Autodesk Inventor part; units mm, degrees
ref_plane "Work Plane1" through (94.25, -2.5, 0) normal (1, 0, 0) x (0, 0, -1)
ref_plane "YZ Plane" through (0, 0, 0) normal (1, 0, 0) x (0, 1, 0)
ref_plane "XZ Plane" through (0, 0, 0) normal (0, 1, 0) x (-1, 0, 0)
sketch "Sketch2" plane through (0, 0, 0) normal (0, 0, 1) x (1, 0, 0)
  line L0 (-99.5, 2.5) -> (99.5, 2.5)
  line L1 (99.5, 2.5) -> (99.5, -2.5)
  line L2 (99.5, -2.5) -> (-99.5, -2.5)
  line L3 (-99.5, -2.5) -> (-99.5, 2.5)
  point P0 (0, 0)
  dimension "d1" = 199
  dimension "d2" = 5
  dimension "d3" = 2.5
  dimension "d4" = 99.5
sketch "Sketch3" plane through (0, 0, 0) normal (1, 0, 0) x (0, 1, 0)
  line L0 (0, 0) -> (-53.033, 53.033)
  line L1 (0, -0.5221) -> (1.6531, -0.5221)
  dimension "d5" = 75
  dimension "d6" = 45
sweep "Sweep1" add profiles "Sketch2" path "Sketch3" path curves L0
sketch "Sketch4" plane through (-99.5, 2.5, 0) normal (0, 0.7071, 0.7071) x (1, 0, 0)
  line L0 (0, 0) -> (199, 0)
  line L1 (0, 0) -> (0, -75)
  line L2 (199, -75) -> (0, -75)
  line L3 (199, 0) -> (199, -75)
  line L4 (199, 0) -> (199, -75)
  line L5 (199, 0) -> (274, -75)
  line L6 (274, -75) -> (199, -75)
  point P0 (99.5, -1.7678)
  dimension "d9" = 45
sketch "Sketch5" plane through (99.5, -2.5, 0) normal (1, 0, 0) x (0, 0, -1)
  line L0 (0, 5) -> (0, 0)
  line L1 (0, 5) -> (-53.033, -48.033)
  line L2 (-53.033, -53.033) -> (-53.033, -48.033)
  line L3 (0, 0) -> (-53.033, -53.033)
  line L4 (-26.5165, -21.5165) -> (-26.5165, -26.5165)
  point P0 (0, 2.5)
sweep "Sweep2" [suppressed]
mirror "Mirror1" [suppressed]
sketch "Sketch6" plane through (99.5, 2.5, 0) normal (0, 0, -1) x (-1, 0, 0)
  line L0 (199, 0) -> (0, 0)
  line L1 (0, 0) -> (0, -5)
  line L2 (0, -5) -> (199, -5)
  line L3 (199, -5) -> (199, 0)
  line L4 (0, 0) -> (199, 0)
  line L5 (199, 0) -> (199, -2)
  line L6 (199, -2) -> (0, -2)
  line L7 (0, -2) -> (0, 0)
  line L8 (98.5, -2) -> (100.5, -2)
  line L9 (100.5, -2) -> (100.5, -5)
  line L10 (100.5, -5) -> (98.5, -5)
  line L11 (98.5, -5) -> (98.5, -2)
  line L12 (48.25, -2) -> (50.25, -2)
  line L13 (50.25, -2) -> (50.25, -5)
  line L14 (50.25, -5) -> (48.25, -5)
  line L15 (48.25, -5) -> (48.25, -2)
  line L16 (148.75, -2) -> (150.75, -2)
  line L17 (150.75, -2) -> (150.75, -5)
  line L18 (150.75, -5) -> (148.75, -5)
  line L19 (148.75, -5) -> (148.75, -2)
  point P0 (99.5, -2.5)
  dimension "d12" = 2
  dimension "d13" = 2
  dimension "d14" = 199
  dimension "d15" = 1
  dimension "d16" = 2
  dimension "d17" = 2
  dimension "d18" = 48.25
  dimension "d19" = 48.25
  dimension "d20" = 48.25
  dimension "d21" = 48.25
extrude "Extrusion1" [suppressed]
sketch "Sketch7" plane through (1, 0.5, 0) normal (0, -1, 0) x (1, 0, 0)
  line L0 (63, 0) -> (63, -10)
  line L1 (124, -10) -> (63, -10)
  line L2 (124, 0) -> (124, -10)
  line L3 (63, 0) -> (124, 0)
  line L4 (61, 0) -> (61, -10)
  line L5 (0, 0) -> (61, 0)
  line L6 (0, 0) -> (0, -10)
  line L7 (61, -10) -> (0, -10)
  line L8 (-63, 0) -> (-63, -10)
  line L9 (-2, -10) -> (-63, -10)
  line L10 (-2, 0) -> (-2, -10)
  line L11 (-63, 0) -> (-2, 0)
  line L12 (-65, -10) -> (-65, 0)
  line L13 (-126, 0) -> (-65, 0)
  line L14 (-126, 0) -> (-126, -10)
  line L15 (-65, -10) -> (-126, -10)
  line L16 (67, -4) -> (57, -4)
  line L17 (57, -4) -> (57, -6)
  line L18 (57, -6) -> (67, -6)
  line L19 (67, -6) -> (67, -4)
  line L20 (4, -4) -> (-6, -4)
  line L21 (-6, -4) -> (-6, -6)
  line L22 (-6, -6) -> (4, -6)
  line L23 (4, -6) -> (4, -4)
  line L24 (-59, -4) -> (-69, -4)
  line L25 (-69, -4) -> (-69, -6)
  line L26 (-69, -6) -> (-59, -6)
  line L27 (-59, -6) -> (-59, -4)
  point P0 (-1, 0)
  dimension "d24" = 10
  dimension "d25" = 2
  dimension "d26" = 4
  dimension "d27" = 4
  dimension "d28" = 4
  dimension "d29" = 4
  dimension "d30" = 10
  dimension "d31" = 2
  dimension "d32" = 4
  dimension "d33" = 4
  dimension "d34" = 4
  dimension "d35" = 10
  dimension "d36" = 4
  dimension "d39" = 2
  dimension "d40" = 4
  dimension "d41" = 4
extrude "Extrusion2" [suppressed]
sketch "Sketch10" plane through (99.5, 2.5, 0) normal (0, 0, -1) x (-1, 0, 0)
  line L0 (199, 0) -> (0, 0)
  line L1 (0, 0) -> (0, -5)
  line L2 (0, -5) -> (199, -5)
  line L3 (199, -5) -> (199, 0)
  line L4 (15, 0) -> (184, 0)
  line L5 (184, 0) -> (184, -2)
  line L6 (184, -2) -> (15, -2)
  line L7 (15, -2) -> (15, 0)
  point P0 (99.5, -2.5)
  dimension "d76" = 2
  dimension "d77" = 169
  dimension "d78" = 84.5
extrude "Extrusion5" add sketch "Sketch10" along normal blind 10 contours L5 L6 L7 L0
sketch "Sketch11" plane through (-84.5, 0.5, 0) normal (0, -1, 0) x (1, 0, 0)
  line L0 (0, 0) -> (169, 0)
  line L1 (0, 0) -> (0, -10)
  line L2 (169, -10) -> (0, -10)
  line L3 (169, 0) -> (169, -10)
  line L4 (149.25, -6) -> (119.25, -6)
  line L5 (119.25, -6) -> (119.25, -4)
  line L6 (119.25, -4) -> (149.25, -4)
  line L7 (149.25, -4) -> (149.25, -6)
  line L8 (99.5, -6) -> (69.5, -6)
  line L9 (69.5, -6) -> (69.5, -4)
  line L10 (69.5, -4) -> (99.5, -4)
  line L11 (99.5, -4) -> (99.5, -6)
  line L12 (49.75, -6) -> (19.75, -6)
  line L13 (19.75, -6) -> (19.75, -4)
  line L14 (19.75, -4) -> (49.75, -4)
  line L15 (49.75, -4) -> (49.75, -6)
  point P0 (84.5, 0)
  dimension "d81" = 2
  dimension "d82" = 10
  dimension "d83" = 4
  dimension "d84" = 30
  dimension "d85" = 19.75
  dimension "d86" = 169
  dimension "d87" = 19.75
  dimension "d88" = 19.75
  dimension "d89" = 30
  dimension "d90" = 30
  dimension "d91" = 19.75
extrude "Extrusion6" add sketch "Sketch11" along normal blind 6 contours L4 L5 L6 L7 | L8 L9 L10 L11 | L12 L13 L14 L15
sketch "Sketch12" plane through (99.5, -2.5, 0) normal (1, 0, 0) x (0, 0, -1)
  line L0 (0, 5) -> (0, 0)
  line L1 (0, 5) -> (-53.033, -48.033)
  line L2 (-53.033, -53.033) -> (-53.033, -48.033)
  line L3 (0, 0) -> (-53.033, -53.033)
  line L4 (-7.0711, -2.0711) -> (-7.0711, -4.5711)
  line L5 (-7.0711, -4.5711) -> (-45.9619, -43.4619)
  line L6 (-45.9619, -43.4619) -> (-45.9619, -40.9619)
  line L7 (-45.9619, -40.9619) -> (-7.0711, -2.0711)
  dimension "d99" = 2.5
  dimension "d100" = 10
  dimension "d101" = 10
extrude "Extrusion7" cut sketch "Sketch12" against normal blind 10.5 contours L4 L5 L6 L1
ref_plane "Work Plane1" through (94.25, -2.5, 0) normal (1, 0, 0) x (0, 0, -1)
sketch "Sketch13" plane through (94.25, -2.5, 0) normal (1, 0, 0) x (0, 0, -1)
  line L0 (-7.0711, -2.0711) -> (-7.0711, -4.5711)
  line L1 (-7.0711, -4.5711) -> (-45.9619, -43.4619)
  line L2 (-45.9619, -43.4619) -> (-45.9619, -40.9619)
  line L3 (-45.9619, -40.9619) -> (-53.033, -48.033)
  line L4 (-53.033, -53.033) -> (-53.033, -48.033)
  line L5 (0, 0) -> (-53.033, -53.033)
  line L6 (0, 5) -> (0, 0)
  line L7 (0, 5) -> (-7.0711, -2.0711)
  line L8 (-45.9619, -40.9619) -> (-7.0711, -2.0711)
  line L9 (-45.9619, -43.4619) -> (-45.9619, -40.9619)
  line L10 (-7.0711, -4.5711) -> (-45.9619, -43.4619)
  line L11 (-7.0711, -2.0711) -> (-7.0711, -4.5711)
  line L12 (-13.0815, -10.5815) -> (-13.0815, -13.0815)
  line L13 (-13.0815, -13.0815) -> (-23.6881, -23.6881)
  line L14 (-23.6881, -23.6881) -> (-23.6881, -21.1881)
  line L15 (-23.6881, -21.1881) -> (-13.0815, -10.5815)
  line L16 (-29.3449, -26.8449) -> (-29.3449, -29.3449)
  line L17 (-29.3449, -29.3449) -> (-39.9515, -39.9515)
  line L18 (-39.9515, -39.9515) -> (-39.9515, -37.4515)
  line L19 (-39.9515, -37.4515) -> (-29.3449, -26.8449)
  point P0 (0, 2.5)
  dimension "d104" = 15
  dimension "d105" = 15
  dimension "d106" = 8.5
  dimension "d107" = 8.5
  dimension "d108" = 8
  dimension "d109" = 55
extrude "Extrusion8" cut sketch "Sketch13" along normal mid plane 3 contours L12 L5 L14 L1 | L1 L16 L5 L18
mirror "Mirror2" about plane through (0, 0, 0) normal (1, 0, 0) of "Extrusion7", "Extrusion8"
ref_plane "Work Plane2" through (-94.25, -2.5, 0) normal (1, 0, 0) x (0, 0, -1)
equation "\"d19\" = d18"
equation "\"d30\" = d24"
equation "\"d31\" = d25"
equation "\"d32\" = d26"
equation "\"d34\" = d27"
equation "\"d35\" = d24"
equation "\"d36\" = d26"
equation "\"d39\" = d25"
equation "\"d41\" = d27"
equation "\"d83\" = -0.5 * d81 + 0.5 * d82"
equation "\"d85\" = -0.75 * d84 + 0.25 * d86"
equation "\"d87\" = d85"
equation "\"d88\" = d85"
equation "\"d89\" = d84"
equation "\"d90\" = d84"
properties part number "Roof Width Extension"
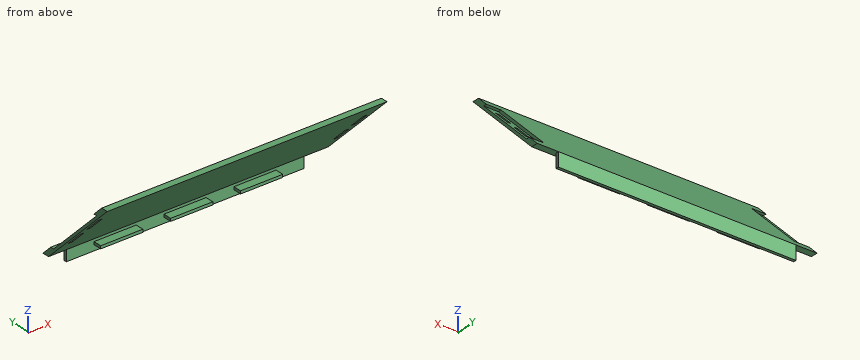
Geometry check sheet. Reference: the model listing, model coordinates, mm. Give positions to 0.01 mm unless a question says otherwise; leave off trailing zeros. Order: outer loops, then holes, each group sorted by start corner. A loop starts at its lowest first (then second) coordinate and runs counter-clockwise, first axis right, second up. Notation, with made-up numbers: (-21.75, -12) - (0.25, -12) arc R27 ccw to (0.25, 12) - close; hole circle Ø7 at (-26, -5). An arc over 180 degrees is marked (long way). Use one line per item in the form item = value.
1) Material ranges on probe 1 along X at (y, z) = (-37, 35); probe 2 along Y at (x, z) = (-52, -6.5); probe 3 along Z at (x, y) = (91.5, -44), recorded low to high. Write a range as from..to.
Working result:
probe_1 = -99.5..-95.75, -92.75..92.75, 95.75..99.5
probe_2 = 0.5..2.5
probe_3 = 41.5..44, 45.96..46.5
2) Sectioned sample at D-D (y = -48). Record the boundary of the cut face in (x, z), and give its area (3 significant figures).
Working result:
outline = (-99.5, 45.5) - (99.5, 45.5) - (99.5, 50.5) - (-99.5, 50.5) - close
area = 995 mm^2
3) Depth check by flat-ended pin: pin 1 Ø5 at (x, z) = (18.5, 39) entering from +Y; pin 2 Ø8 at (x, z) = (-10, 46.5) entering from -Y; pin 3 Ø2 at (x, z) = (-1.5, -5.5) entering from -Y. Enter the tip coordinate at first touch or a pass-through.
Working result:
pin_1 = -34
pin_2 = -53
pin_3 = -5.5
4) Sectioned sample at A-A (y = -35.5). Record the boundary of the cut face in (x, z), and give its area (4 significant figures).
Working result:
outline = (-99.5, 33) - (-95.75, 33) - (-95.75, 35.5) - (-99.5, 35.5) - close; (-92.75, 33) - (92.75, 33) - (92.75, 35.5) - (89, 35.5) - (89, 38) - (-89, 38) - (-89, 35.5) - (-92.75, 35.5) - close; (95.75, 33) - (99.5, 33) - (99.5, 35.5) - (95.75, 35.5) - close
area = 927.5 mm^2
5) Sectioned sample at C-C (x = 17). Record the boundary of the cut face in (y, z).
Working result:
outline = (-55.53, 53.03) - (-2.5, 0) - (0.5, 0) - (0.5, -10) - (2.5, -10) - (2.5, 0) - (-50.53, 53.03) - close
6) Sectioned sample at B-B (z = 33). Record the boundary of the cut face in (x, y).
Working result:
outline = (-99.5, -35.5) - (-95.75, -35.5) - (-95.75, -33) - (-99.5, -33) - close; (-92.75, -35.5) - (92.75, -35.5) - (92.75, -33) - (89, -33) - (89, -30.5) - (-89, -30.5) - (-89, -33) - (-92.75, -33) - close; (95.75, -35.5) - (99.5, -35.5) - (99.5, -33) - (95.75, -33) - close
